Model file for the job. Use its own axes, mm. Face numbers are marked on the shaded views. Round coordinates to 2 decimals unless told otherwise and drop trailing zeros. Order: outer loops, then holes, each group sorted by start corner. A loop starts at its lowest first (then second) coordinate and runs counter-clockwise, first axis right, second up. Notation, with made-up numbers: (-17.75, 13.5) - (9.25, 13.5) arc R23 cw to (9.25, 25.5) - close; hole circle Ø5 at (67, 3). An arc over 180 degrees is marked (long way). Use one line per item in the form item = value.
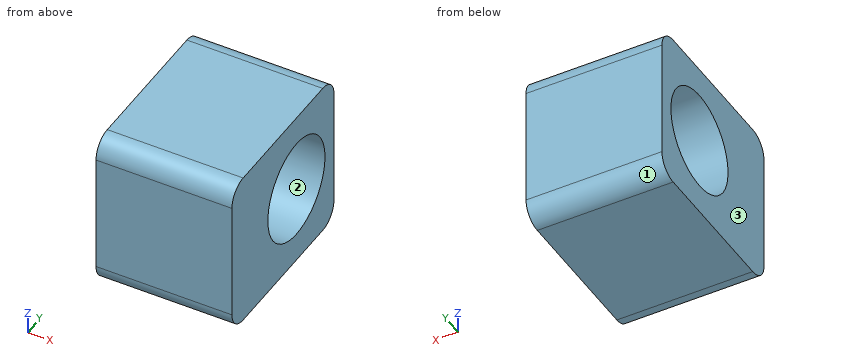
from build123d import *

# Parameters (mm, degrees)
SKETCH1_R           = 12.7
BOSS_EXTRUDE1_DEPTH = 17


with BuildPart() as part:
    # Sketch1 → Boss-Extrude1 (new, symmetric)
    with BuildSketch(Plane(origin=(0, 0, 0), x_dir=(0, 0, -1), z_dir=(1, 0, 0))):
        with BuildLine():
            Line((-15, -28.7), (15, -28.7))
            ThreePointArc((15, -28.7), (18.535533906, -27.235533906), (20, -23.7))
            Line((20, -23.7), (20, 11.7))
            ThreePointArc((20, 11.7), (18.535533906, 15.235533906), (15, 16.7))
            Line((15, 16.7), (-15, 16.7))
            ThreePointArc((-15, 16.7), (-18.535533906, 15.235533906), (-20, 11.7))
            Line((-20, 11.7), (-20, -23.7))
            ThreePointArc((-20, -23.7), (-18.535533906, -27.235533906), (-15, -28.7))
        make_face()
        Circle(SKETCH1_R, mode=Mode.SUBTRACT)
    extrude(amount=BOSS_EXTRUDE1_DEPTH, both=True)


solid = part.part
(1) Slice it at B-B on y = 0. Give the cut face in (x, z), then the cut area to 3 significant figures.
Report:
outline = (-17, -20) - (17, -20) - (17, -12.7) - (-17, -12.7) - close; (-17, 12.7) - (17, 12.7) - (17, 20) - (-17, 20) - close
area = 496 mm2
(2) Slice it at C-C on x = -5.5. Give the cut face in (y, z), then the cut area to 3 significant figures.
Report:
outline = (-28.7, -15) arc R5 ccw to (-23.7, -20) - (11.7, -20) arc R5 ccw to (16.7, -15) - (16.7, 15) arc R5 ccw to (11.7, 20) - (-23.7, 20) arc R5 ccw to (-28.7, 15) - close; hole circle Ø25.4 at (0, 0)
area = 1,290 mm2
(3) Slice it at D-D on y = 13.5. Give the cut face in (x, z), then the cut area to 3 significant figures.
Report:
outline = (-17, -19.66) - (17, -19.66) - (17, 19.66) - (-17, 19.66) - close
area = 1,340 mm2
(4) Pull direction Y, two halves, no side cores. Call the marked faces 1, 2 and 3: released by +Y, released by -Y, zero draft, split by the parting line, or undercut.
Report:
face_1 = released by +Y
face_2 = undercut
face_3 = zero draft
(5) Probe probe 1 along Y at (x, z) = (2, 0); probe 2 along Y at (x, z) = (-1.5, 7); probe 3 along Z at (x, y) = (-13, 7). List the from-to ranges inside material, lowest first. Write a range as [from, to].
Report:
probe_1 = [-28.7, -12.7], [12.7, 16.7]
probe_2 = [-28.7, -10.6], [10.6, 16.7]
probe_3 = [-20, -10.6], [10.6, 20]
(6) Slice it at A-A on z = 0. Give the cut face in (x, y), then the cut area to 3 significant figures.
Report:
outline = (-17, -28.7) - (17, -28.7) - (17, -12.7) - (-17, -12.7) - close; (-17, 12.7) - (17, 12.7) - (17, 16.7) - (-17, 16.7) - close
area = 680 mm2
